Verification items for the finished model (mm, model axes). Face numbers are marked on the shaded views. A direction names the side the tool comes from. Round coordinates to 2 decimals unless told otherwise and drop trailing zeros. Order: outer loops, then holes, each group sorted by start corner. A loop starts at its lowest first (then second) coordinate and runs counter-clockwise, first axis right, second up. Notation, with made-up numbers: M 81,41 L 97,41 A35 ccw 97,76 Z; hole C -15.75,82 d1. An arc over 180 degrees is marked long. Use CSV: the item, a comma, the result in double quotes. Start each with the question number.
Q1. Sectioned sample at C-C (z = -60). Enter the section's corners in (x, y).
Q2. Set-up check for the marked faces 1 and 2: record each of +Z, -Z, +X, -X, +Y, -Y from which the full face is reachable in a straight line by a thin tool's end or side.
Q3. Sectioned sample at D-D (x = 39). Enter the section's corners in (y, z).
Q4. Sectioned sample at B-B (x = 90). Enter the section's corners in (y, z).
Q5. Mould release check, pull along Y, two halves, no side actions. Record for the marked faces 3, 4 and 5: +Y half, -Y half, draft (parallel to the pull), parting line (faces both ways), or undercut.
Q6. Sectioned sample at A-A (y = -89.5). Enter the section's corners in (x, z).
Q7. Gauge pin test, flat ends, axial feed: pin 1 Ø7 at (x, y) = (30.5, 453) entering from +Z; pin 2 Ø2 at (y, z) = (-62.5, 136) entering from +X; pin 3 Ø6 at (y, z) = (-151.5, 176) entering from -X. Record the tip position at first contact, or that the pin passes through.
Q8. Scan lines: line 1 (Y direction, x = 72.5, z = -73); line 2 (Z direction, x = 7.5, y = -197); line 3 (Z direction, x = 39, y = 233). Record each from-to range of solid material in increasing order.
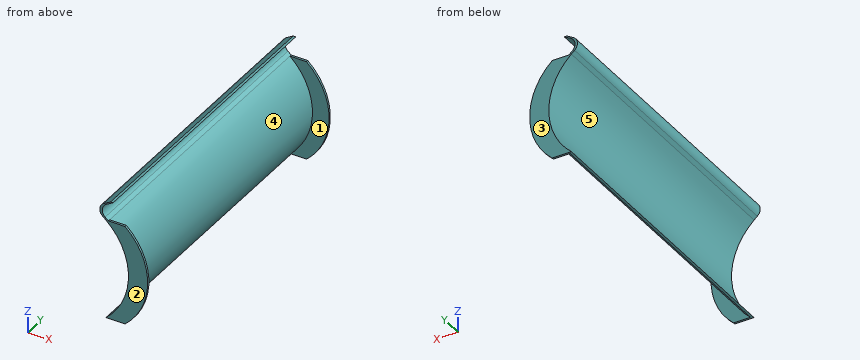
```python
from build123d import *

# Parameters (mm, degrees)
F1_DEPTH = 457.2
F3_DEPTH = 6.35


with BuildPart() as f1:
    # F0 (on Front) → F1 (new body, symmetric)
    with BuildSketch(Plane.XZ):
        with BuildLine():
            Line((-7.632641, -152.4), (0, -152.4))
            ThreePointArc((0, -152.4), (68.795833, 0), (0, 152.4))
            Line((0, 152.4), (-9.967424, 160.932384))
            ThreePointArc((-9.967424, 160.932384), (-18.7435, 182.548823), (-6.180466, 202.207412))
            Line((-6.180466, 202.207412), (13.96697, 213.877112))
            Line((13.96697, 213.877112), (6.334329, 213.877112))
            Line((6.334329, 213.877112), (-13.813108, 202.207412))
            ThreePointArc((-13.813108, 202.207412), (-26.376141, 182.548823), (-17.600065, 160.932384))
            Line((-17.600065, 160.932384), (-7.632641, 152.4))
            ThreePointArc((-7.632641, 152.4), (61.163192, 0), (-7.632641, -152.4))
        make_face()
    extrude(amount=F1_DEPTH, both=True)

    # F2 (on face) → F3 (join)
    with BuildSketch(Plane.XZ.offset(457.2)):
        with BuildLine():
            Line((50.8, 152.4), (0, 152.4))
            ThreePointArc((0, 152.4), (68.795833, 0), (0, -152.4))
            Line((0, -152.4), (50.8, -152.4))
            ThreePointArc((50.8, -152.4), (119.595833, 0), (50.8, 152.4))
        make_face()
    extrude(amount=-F3_DEPTH)

    # F4: F1 across plane


with BuildPart() as f1_1:
    add(f1.part)
    add(f1.part.mirror(Plane.XZ))


solid = f1_1.part
```
Verdict:
1,outline,"M 52.1,-457.2 L 110.54,-457.2 L 110.54,-450.85 L 59.74,-450.85 L 59.74,450.85 L 110.54,450.85 L 110.54,457.2 L 52.1,457.2 Z"
2,face 1,"+X"
2,face 2,"+Z, -Z, +X, -X, -Y"
3,outline,"M -457.2,-152.4 L -450.85,-152.4 L -450.85,-105.93 L 450.85,-105.93 L 450.85,-152.4 L 457.2,-152.4 L 457.2,-92.28 L -457.2,-92.28 Z; M -457.2,92.28 L 457.2,92.28 L 457.2,152.4 L 450.85,152.4 L 450.85,105.93 L -450.85,105.93 L -450.85,152.4 L -457.2,152.4 Z"
4,outline,"M -457.2,-105.6 L -450.85,-105.6 L -450.85,105.6 L -457.2,105.6 Z; M 450.85,-105.6 L 457.2,-105.6 L 457.2,105.6 L 450.85,105.6 Z"
5,face 3,"+Y half"
5,face 4,"undercut"
5,face 5,"draft"
6,outline,"M -17.6,160.93 L -7.63,152.4 A203.2 cw -7.63,-152.4 L 0,-152.4 A203.2 ccw 0,152.4 L -9.97,160.93 A25.4 cw -6.18,202.21 L 13.97,213.88 L 6.33,213.88 L -13.81,202.21 A25.4 ccw Z"
7,pin 1,"stops at z = 152.4"
7,pin 2,"stops at x = 17.47"
7,pin 3,"stops at x = -26.45"
8,line 1,"y = -457.2 to -450.85, 450.85 to 457.2"
8,line 2,"z = -145.44 to -137.58, 137.58 to 145.44, 210.13 to 213.88"
8,line 3,"z = -105.93 to -92.28, 92.28 to 105.93"
